```python
from build123d import *

# Parameters (mm, degrees)
BOSS_EXTRUDE1_DEPTH = 0.7
SKETCH5_R           = 5
CUT_EXTRUDE1_DEPTH  = 27
SKETCH6_R           = 5
CUT_EXTRUDE2_DEPTH  = 27


with BuildPart() as part:
    # Sketch2 → Boss-Extrude1 (new body)
    with BuildSketch(Plane.XY):
        with BuildLine():
            Line((-20.5, -0.35), (-13.5, -0.35))
            ThreePointArc((-13.5, -0.35), (-12.545405845, 0.045405845), (-12.15, 1))
            Line((-12.15, 1), (-12.15, 7))
            ThreePointArc((-12.15, 7), (-11, 8.15), (-9.85, 7))
            Line((-9.85, 7), (-9.85, 0))
            Line((-9.85, 0), (-9.85, -7))
            ThreePointArc((-9.85, -7), (-8, -8.85), (-6.15, -7))
            Line((-6.15, -7), (-6.15, 0))
            Line((-6.15, 0), (-6.15, 7))
            ThreePointArc((-6.15, 7), (-5, 8.15), (-3.85, 7))
            Line((-3.85, 7), (-3.85, 0))
            Line((-3.85, 0), (-3.85, -7))
            ThreePointArc((-3.85, -7), (-2, -8.85), (-0.15, -7))
            Line((-0.15, -7), (-0.15, 0))
            Line((-0.15, 0), (-0.15, 7))
            ThreePointArc((-0.15, 7), (1, 8.15), (2.15, 7))
            Line((2.15, 7), (2.15, 0))
            Line((2.15, 0), (2.15, -7))
            ThreePointArc((2.15, -7), (4, -8.85), (5.85, -7))
            Line((5.85, -7), (5.85, -1))
            ThreePointArc((5.85, -1), (6.040380592, -0.540380592), (6.5, -0.35))
            Line((6.5, -0.35), (13.5, -0.35))
            ThreePointArc((13.5, -0.35), (13.85, 0), (13.5, 0.35))
            Line((13.5, 0.35), (6.5, 0.35))
            ThreePointArc((6.5, 0.35), (5.545405845, -0.045405845), (5.15, -1))
            Line((5.15, -1), (5.15, -7))
            ThreePointArc((5.15, -7), (4, -8.15), (2.85, -7))
            Line((2.85, -7), (2.85, 0))
            Line((2.85, 0), (2.85, 7))
            ThreePointArc((2.85, 7), (1, 8.85), (-0.85, 7))
            Line((-0.85, 7), (-0.85, 0))
            Line((-0.85, 0), (-0.85, -7))
            ThreePointArc((-0.85, -7), (-2, -8.15), (-3.15, -7))
            Line((-3.15, -7), (-3.15, 0))
            Line((-3.15, 0), (-3.15, 7))
            ThreePointArc((-3.15, 7), (-5, 8.85), (-6.85, 7))
            Line((-6.85, 7), (-6.85, 0))
            Line((-6.85, 0), (-6.85, -7))
            ThreePointArc((-6.85, -7), (-8, -8.15), (-9.15, -7))
            Line((-9.15, -7), (-9.15, 0))
            Line((-9.15, 0), (-9.15, 7))
            ThreePointArc((-9.15, 7), (-11, 8.85), (-12.85, 7))
            Line((-12.85, 7), (-12.85, 1))
            ThreePointArc((-12.85, 1), (-13.040380592, 0.540380592), (-13.5, 0.35))
            Line((-13.5, 0.35), (-20.5, 0.35))
            ThreePointArc((-20.5, 0.35), (-20.85, 0), (-20.5, -0.35))
        make_face()
    extrude(amount=BOSS_EXTRUDE1_DEPTH)

    # Sketch3 → Revolve1 (revolve)
    with BuildSketch(Plane(origin=(0, 0, 0), x_dir=(1, 0, 0), z_dir=(0, 1, 0)), mode=Mode.PRIVATE) as revolve1_sk:
        Polygon((-20.5, -0.7), (-25.5, -0.7), (-26.5, 3.3), (-26.5, 29.3), (-20.5, 29.3), align=None)
    revolve(revolve1_sk.sketch.rotate(Axis((-20.5, 0, 0.7), (0, 0, -1)), 175.986012782), axis=Axis((-20.5, 0, 0.7), (0, 0, -1)))

    # Sketch4 → Revolve2 (revolve)
    with BuildSketch(Plane(origin=(0, 0, 0), x_dir=(1, 0, 0), z_dir=(0, 1, 0)), mode=Mode.PRIVATE) as revolve2_sk:
        Polygon((13.5, -0.69956823), (18.5, -0.69956823), (19.5, 3.30043177), (19.5, 29.30043177), (13.5, 29.30043177), align=None)
    revolve(revolve2_sk.sketch.rotate(Axis((13.5, 0, 0.69956823), (0, 0, -1)), 176.121883858), axis=Axis((13.5, 0, 0.69956823), (0, 0, -1)))

    # Sketch5 → Cut-Extrude1 (cut)
    with BuildSketch(Plane(origin=(0, 0, -29.3), x_dir=(-1, 0, 0), z_dir=(0, 0, -1))):
        with Locations((-13.5, 0)):
            Circle(SKETCH5_R)
        with Locations((20.5, 0)):
            Circle(SKETCH5_R)
    extrude(amount=-CUT_EXTRUDE1_DEPTH, mode=Mode.SUBTRACT)

    # Sketch6 → Cut-Extrude2 (cut)
    with BuildSketch(Plane(origin=(0, 0, -29.30043177), x_dir=(-1, 0, 0), z_dir=(0, 0, -1))):
        with Locations((-13.5, 0)):
            Circle(SKETCH6_R)
    extrude(amount=-CUT_EXTRUDE2_DEPTH, mode=Mode.SUBTRACT)


solid = part.part
```
Could you check a few things on this model? Use its own coordinates, in mm. A direction names the side the tool comes from. Coordinates: 2 decimals unless noted, no trailing zeros. Write each loop counter-clockwise with the first axis right and the second up, starting at its lowest first coordinate (ties: lowest second). Pieces come first, ordered by that corner, then holes. Notation, with made-up numbers: (66, 6.5) - (125, 6.5) arc R23 cw to (125, 40.5) - close; hole circle Ø4 at (-16.75, 86). An arc over 180 degrees is marked (long way). Use a Markdown table: item, result.
Q1. Imagine slicing it at B-B (z = -23). List the corners of the cut face in (x, y) for me.
Geometry check:
| item | result |
|---|---|
| outline | circle Ø12 at (-20.5, 0); circle Ø12 at (13.5, 0); hole circle Ø10 at (-20.5, 0); hole circle Ø10 at (13.5, 0) |
Q2. Imagine slicing it at A-A (x = -20.5). List the corners of the cut face in (y, z) for me, and give its area (3 significant figures).
Geometry check:
| item | result |
|---|---|
| outline | (-6, -29.3) - (-5, -29.3) - (-5, -2.3) - (5, -2.3) - (5, -29.3) - (6, -29.3) - (6, -3.3) - (5, 0.7) - (-5, 0.7) - (-6, -3.3) - close |
| area | 86.0 mm2 |
Q3. Which directions (+Z, -Z, +X, -X, +Y, -Y) give clear straight access to the entire face, cutting with the end or side of a thin tool? Please do faces 1 (the cylindrical face through (5.56, -0.03, 0.35)), 2 (the flat face through (14, 0, -2.3)), 3 (the cylindrical face through (-8.04, -8.85, 0.35)).
Geometry check:
| item | result |
|---|---|
| face 1 | +Z, -Z, +Y |
| face 2 | -Z |
| face 3 | +Z, -Z, -Y |
Q4. Imagine slicing it at C-C (y = 1.5). Count the separate pieces of the cut face and the enclosed holes in it, and give its area (3 significant figures).
Geometry check:
| item | result |
|---|---|
| separate pieces | 8 |
| enclosed holes | 0 |
| area | 177 mm2 |
Q5. I'm going to push flat-ended pins straight in: pin 1 Ø0.8 at (y, z) = (-2.5, 0.5) entering from +X; pin 2 Ø0.8 at (x, z) = (9.5, 0.5) entering from -Y; pin 3 Ø0.8 at (y, z) = (-3, 0.5) entering from -X. Where does each tip first touch, or does it pass through?
Geometry check:
| item | result |
|---|---|
| pin 1 | stops at x = 18.12 |
| pin 2 | stops at y = -3.57 |
| pin 3 | stops at x = -24.86 |
Q6. Please list where these lines run through material, in increasing order: L1, parallel to X at y = 0.25, z = -20; L2, parallel to Y at x = 13.5, z = -17; L3, parallel to X at y = -0.25, z = -2.5.
Geometry check:
| item | result |
|---|---|
| L1 | x = -26.49 to -25.49, -15.51 to -14.51, 7.51 to 8.51, 18.49 to 19.49 |
| L2 | y = -6 to -5, 5 to 6 |
| L3 | x = -26.29 to -25.49, -15.51 to -14.71, 7.71 to 8.51, 18.49 to 19.29 |
Q7. Thinking about a two-plate mould opening in Y: for faces 4 (the cylindrical face through (-10.96, 8.85, 0.35)), 5 (the flat face through (-20, 0, -2.3)), 6 (the cylindrical face through (-2.04, -8.85, 0.35)), 7 (the flat face through (15, 5, -29.3)), which applies, +Y half, -Y half, draft (parallel to the pull), parting line (faces both ways), or undercut?
Geometry check:
| item | result |
|---|---|
| face 4 | +Y half |
| face 5 | undercut |
| face 6 | -Y half |
| face 7 | draft |
